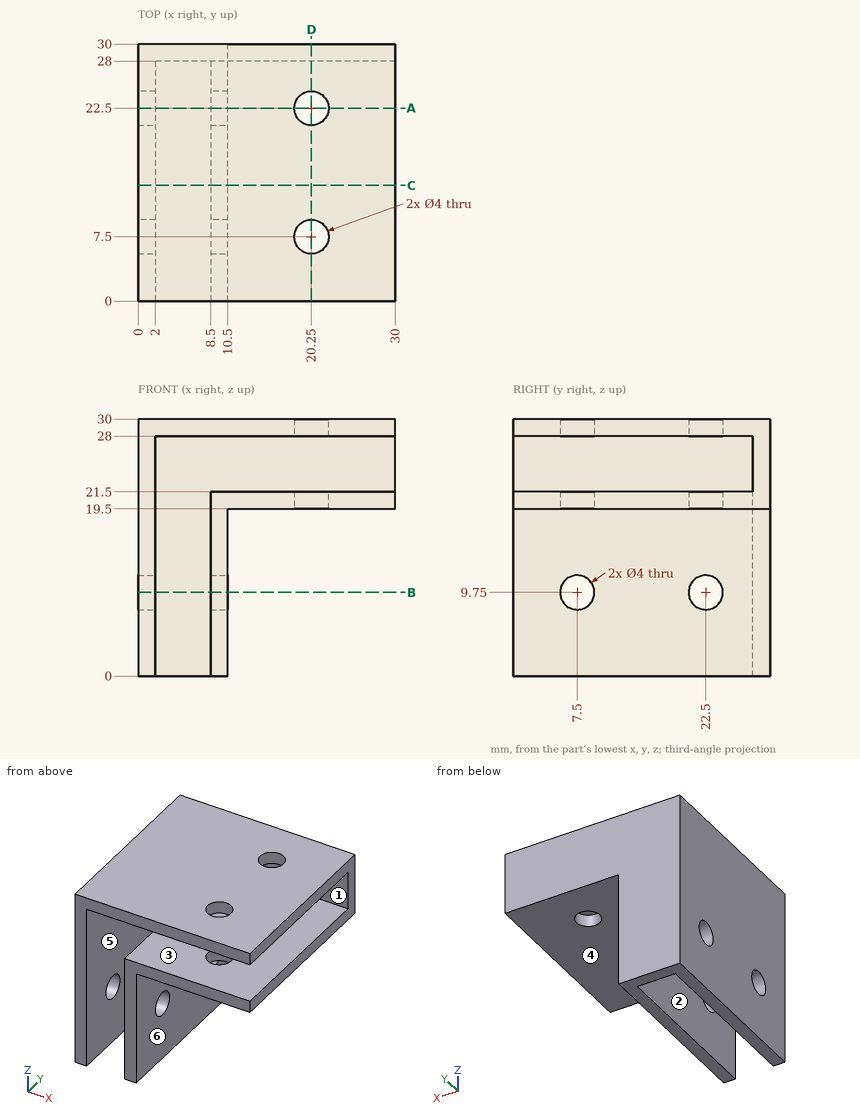
Source: three-view drawing plus pictorial views. Frame: mm from the lowest corner of the part. A direction names the side the tool comes from. Round coordinates to 2 decimals unless told otherwise and drop trailing zeros. Loops run counter-clockwise (first coordinate to the right, second up) from the corner with the lowest first, then second, coordinate; pieces in that order, holes last. Notation, with made-up numbers: M 33.5,33.25 L 60.5,33.25 A20 ccw 60.5,62.25 Z; hole C 27,57 d2. An arc over 180 degrees is marked long. Put each result on its own line as item: value.
(1) First-contact query: pin 1 (1.5 mm diameter, centred on x = 12, y = 16.5, fed in from -Z); pin 2 (12 mm diameter, centred on y = 10.5, z = 5, fed in from +X). Flat tips, straight axial feed; report the tip coordinate or a pass-through.
Solutions:
pin 1: z = 19.5
pin 2: x = 10.5
(2) Access query for the marked faces 1, 2 and 3. Directions: +Z, -Z, +X, -X, +Y, -Y. A direction counts if a zero-diameter tool reaches every point of the face in a straight line with its end or side. Return the directions, or none.
Solutions:
face 1: -Y
face 2: -Z, -Y
face 3: +X, -Y
(3) Pull-direction query (X, two-part tool) for the marked faces 4, 5 and 6; classes: released by +X, released by -X, zero draft, split by the parting line, or undercut.
Solutions:
face 4: zero draft
face 5: undercut
face 6: released by +X
(4) Section A-A, the plane y = 22.5. Return loops of the section in (x, z), and give its area (3 significant figures).
Solutions:
outline: M 0,0 L 2,0 L 2,7.75 L 0,7.75 Z; M 0,11.75 L 2,11.75 L 2,28 L 18.25,28 L 18.25,30 L 0,30 Z; M 8.5,0 L 10.5,0 L 10.5,7.75 L 8.5,7.75 Z; M 8.5,11.75 L 10.5,11.75 L 10.5,19.5 L 18.25,19.5 L 18.25,21.5 L 8.5,21.5 Z; M 22.25,19.5 L 30,19.5 L 30,21.5 L 22.25,21.5 Z; M 22.25,28 L 30,28 L 30,30 L 22.25,30 Z
area: 166 mm²
(5) Section D-D, the plane x = 20.25. Return loops of the section in (y, z).
Solutions:
outline: M 0,19.5 L 5.5,19.5 L 5.5,21.5 L 0,21.5 Z; M 0,28 L 5.5,28 L 5.5,30 L 0,30 Z; M 9.5,19.5 L 20.5,19.5 L 20.5,21.5 L 9.5,21.5 Z; M 9.5,28 L 20.5,28 L 20.5,30 L 9.5,30 Z; M 24.5,19.5 L 30,19.5 L 30,30 L 24.5,30 L 24.5,28 L 28,28 L 28,21.5 L 24.5,21.5 Z
(6) Ray query, line 1 (Y direction, x = 20.25, z = 20.95); line 2 (Z direction, x = 9.35, y = 22.5); line 3 (X direction, y = 15.75, z = 1.5). Return the intervals inside material, ascending. Write a range as [from, to].
Solutions:
line 1: [0, 5.5], [9.5, 20.5], [24.5, 30]
line 2: [0, 7.75], [11.75, 21.5], [28, 30]
line 3: [0, 2], [8.5, 10.5]
(7) Section C-C, the plane y = 13.5. Return loops of the section in (x, z), and give its area (3 significant figures).
Solutions:
outline: M 0,0 L 2,0 L 2,28 L 30,28 L 30,30 L 0,30 Z; M 8.5,0 L 10.5,0 L 10.5,19.5 L 30,19.5 L 30,21.5 L 8.5,21.5 Z
area: 198 mm²
(8) Section B-B, the plane z = 9.75. Return loops of the section in (x, y).
Solutions:
outline: M 0,0 L 2,0 L 2,5.5 L 0,5.5 Z; M 0,9.5 L 2,9.5 L 2,20.5 L 0,20.5 Z; M 0,24.5 L 2,24.5 L 2,28 L 8.5,28 L 8.5,24.5 L 10.5,24.5 L 10.5,30 L 0,30 Z; M 8.5,0 L 10.5,0 L 10.5,5.5 L 8.5,5.5 Z; M 8.5,9.5 L 10.5,9.5 L 10.5,20.5 L 8.5,20.5 Z
